Read the model definition and answer for the solid it produces. Units are mm, in the model's axes. A direction names the side the tool comes from. Coordinates: 2 decimals unless noted, no trailing zeros. Write each loop counter-clockwise with the first axis right and the second up, starting at its lowest first coordinate (ties: lowest second). Pieces come first, ordered by that corner, then holes.
(1) Section D-D on z = 3 is taken. Write down the section's boundary in (x, y), then the cut area to 3 significant figures.
(2) Which of the six approach directions +Z, -Z, +X, -X, +Y, -Y give full straight-line access (tool end or side, diameter ignored) to faces 1 (the flat face through (66.01, 25.51, 26.07)), 2 (the flat face through (-65.99, 25.49, 26.06)), 3 (the flat face through (-66.4, 2.74, 28.52))?
(3) Section A-A on y = 15 is taken. Write down the section's boundary in (x, z).
(4) Section C-C on z = 43.5 is taken. Write down the section's boundary in (x, y), then the cut area to 3 significant figures.
(5) Find the intervals of material crossed by probe 1 along X at (y, z) = (15, -10); probe 2 along Y at (x, z) = (-61, 7.5); probe 3 along Y at (x, z) = (-64.25, -5.5), in increasing order.
(6) Section B-B on x = -64.25 is taken. Write down the section's boundary in (y, z), then the cut area to 3 significant figures.
(7) Given pin 1 (5 mm diameter, centred on x = 43.5, y = 26.5, fed in from +Z); pin 2 (1 mm diameter, centred on y = 16.5, z = 40, fed in from -X); pin 3 (4 mm diameter, centred on x = -6, y = 14, fed in from +Z), each flat-ended and moving along its own axis, determine where each tip first touches the part or whether it passes through.
(8) The mould has two halves that part along X. Classify faces 4 (the flat face through (-66.54, 0.99, 23.92)), 5 (the flat face through (66.4, 27.24, 28.52)), 6 (the flat face through (62, 5.5, 19)), 7 (the cylindrical face through (59.492, 15.209, -7.556)): +X half, -X half, draft (parallel to the pull), parting line (faces both ways), or undercut.
from build123d import *

# Parameters (mm, degrees)
BOSS_EXTRUDE1_DEPTH     = 30
CUT_EXTRUDE2_DEPTH      = 100.544588
CUT_EXTRUDE2_DEPTH_BACK = 100.544588
SKETCH8_R               = 4.7625
SKETCH9_W               = 19
SKETCH9_H               = 5.5
BOSS_EXTRUDE3_DEPTH     = 59.75
CUT_EXTRUDE3_DEPTH      = 98.483973042
CUT_EXTRUDE3_DEPTH_BACK = 98.483973042
CHAMFER4_SIZE           = 2
FILLET2_R               = 2


with BuildPart() as part:
    # Sketch1 → Boss-Extrude1 (new body)
    with BuildSketch(Plane(origin=(0, 0, 0), x_dir=(1, 0, 0), z_dir=(0, 1, 0))):
        with BuildLine():
            Line((-54.75, -11.5), (-54.75, -56.25))
            Line((-54.75, -56.25), (-44.75, -56.25))
            ThreePointArc((-44.75, -56.25), (0, -11.5), (44.75, -56.25))
            Line((44.75, -56.25), (54.75, -56.25))
            Line((54.75, -56.25), (54.75, -11.5))
            Line((54.75, -11.5), (54.75, 3.5))
            Line((54.75, 3.5), (73.75, 3.5))
            Line((73.75, 3.5), (73.75, 11.5))
            Line((73.75, 11.5), (54.75, 11.5))
            Line((54.75, 11.5), (-54.75, 11.5))
            Line((-54.75, 11.5), (-73.75, 11.5))
            Line((-73.75, 11.5), (-73.75, 3.5))
            Line((-73.75, 3.5), (-54.75, 3.5))
            Line((-54.75, 3.5), (-54.75, -11.5))
        make_face()
    extrude(amount=BOSS_EXTRUDE1_DEPTH)

    # Sketch8 → Cut-Extrude2 (cut, two sides: drawn at the far end of the back side and taken through both)
    with BuildSketch(Plane.XY.offset(-3.5).offset(-CUT_EXTRUDE2_DEPTH_BACK)):
        with Locations((-64.25, 15)):
            Circle(SKETCH8_R)
        with Locations((64.25, 15)):
            Circle(SKETCH8_R)
    extrude(amount=CUT_EXTRUDE2_DEPTH + CUT_EXTRUDE2_DEPTH_BACK, mode=Mode.SUBTRACT)

    # Sketch9 → Boss-Extrude3 (add)
    with BuildSketch(Plane.XY.offset(-3.5)):
        with Locations((-64.25, 27.25)):
            Rectangle(SKETCH9_W, SKETCH9_H)
        with Locations((-64.25, 2.75)):
            Rectangle(SKETCH9_W, SKETCH9_H)
        with Locations((64.25, 27.25)):
            Rectangle(SKETCH9_W, SKETCH9_H)
        with Locations((64.25, 2.75)):
            Rectangle(SKETCH9_W, SKETCH9_H)
    extrude(amount=BOSS_EXTRUDE3_DEPTH)

    # Sketch10 → Cut-Extrude3 (cut, two sides: drawn at the far end of the back side and taken through both)
    with BuildSketch(Plane(origin=(0, 30, 0), x_dir=(1, 0, 0), z_dir=(0, 1, 0)).offset(-CUT_EXTRUDE3_DEPTH_BACK)):
        Polygon((-59.25, -56.25), (-73.75, 0), (-73.75, -56.25), align=None)
        Polygon((73.75, -56.25), (59.25, -56.25), (73.75, 0), align=None)
    extrude(amount=CUT_EXTRUDE3_DEPTH + CUT_EXTRUDE3_DEPTH_BACK, mode=Mode.SUBTRACT)

    # Chamfer4
    chamfer4_edges = [part.edges().sort_by_distance(p)[0] for p in [
        (-66.5, 24.5, 28.125),
    ]]
    chamfer(chamfer4_edges, length=CHAMFER4_SIZE)
    chamfer4_2_edges = [part.edges().sort_by_distance(p)[0] for p in [
        (-66.5, 5.5, 28.125),
    ]]
    chamfer(chamfer4_2_edges, length=CHAMFER4_SIZE)
    chamfer4_3_edges = [part.edges().sort_by_distance(p)[0] for p in [
        (-66.5, 0, 28.125),
    ]]
    chamfer(chamfer4_3_edges, length=CHAMFER4_SIZE)
    chamfer4_4_edges = [part.edges().sort_by_distance(p)[0] for p in [
        (66.5, 0, 28.125),
    ]]
    chamfer(chamfer4_4_edges, length=CHAMFER4_SIZE)
    chamfer4_5_edges = [part.edges().sort_by_distance(p)[0] for p in [
        (-66.5, 30, 28.125),
    ]]
    chamfer(chamfer4_5_edges, length=CHAMFER4_SIZE)
    chamfer4_6_edges = [part.edges().sort_by_distance(p)[0] for p in [
        (66.5, 30, 28.125),
    ]]
    chamfer(chamfer4_6_edges, length=CHAMFER4_SIZE)
    chamfer4_7_edges = [part.edges().sort_by_distance(p)[0] for p in [
        (66.5, 5.5, 28.125),
    ]]
    chamfer(chamfer4_7_edges, length=CHAMFER4_SIZE)
    chamfer4_8_edges = [part.edges().sort_by_distance(p)[0] for p in [
        (66.5, 24.5, 28.125),
    ]]
    chamfer(chamfer4_8_edges, length=CHAMFER4_SIZE)

    # Fillet2
    fillet2_edges = [part.edges().sort_by_distance(p)[0] for p in [
        (44.75, 15, 56.25),
        (-44.75, 15, 56.25),
    ]]
    fillet(fillet2_edges, radius=FILLET2_R)


solid = part.part
Response:
1. outline: (-72.98, 2) - (-70.91, 0) - (70.91, 0) - (72.98, 2) - (72.98, 3.5) - (70.91, 5.5) - (54.75, 5.5) - (54.75, 24.5) - (70.91, 24.5) - (72.98, 26.5) - (72.98, 28) - (70.91, 30) - (-70.91, 30) - (-72.98, 28) - (-72.98, 26.5) - (-70.91, 24.5) - (-54.75, 24.5) - (-54.75, 5.5) - (-70.91, 5.5) - (-72.98, 3.5) - close
1. area: 3,670 mm2
2. face 1: +Z, +X
2. face 2: +Z, -X
2. face 3: +Z, -X, +Y, -Y
3. outline: (-73.75, -11.5) - (-69.01, -11.5) - (-69.01, -3.5) - (-73.75, -3.5) - close; (-59.49, -11.5) - (59.49, -11.5) - (59.49, -3.5) - (54.75, -3.5) - (54.75, 56.25) - (46.71, 56.25) arc R2 ccw to (44.71, 54.34) arc R44.75 cw to (-44.71, 54.34) arc R2 ccw to (-46.71, 56.25) - (-54.75, 56.25) - (-54.75, -3.5) - (-59.49, -3.5) - close; (69.01, -11.5) - (73.75, -11.5) - (73.75, -3.5) - (69.01, -3.5) - close
4. outline: (-62.54, 2) - (-60.47, 0) - (-42.9, 0) - (-42.9, 30) - (-60.47, 30) - (-62.54, 28) - (-62.54, 26.5) - (-60.47, 24.5) - (-54.75, 24.5) - (-54.75, 5.5) - (-60.47, 5.5) - (-62.54, 3.5) - close; (42.9, 0) - (60.47, 0) - (62.54, 2) - (62.54, 3.5) - (60.47, 5.5) - (54.75, 5.5) - (54.75, 24.5) - (60.47, 24.5) - (62.54, 26.5) - (62.54, 28) - (60.47, 30) - (42.9, 30) - close
4. area: 866 mm2
5. probe 1: x = -73.75 to -69.01, -59.49 to 59.49, 69.01 to 73.75
5. probe 2: y = 0 to 5.5, 24.5 to 30
5. probe 3: y = 0 to 10.24, 19.76 to 30
6. outline: (0, -11.5) - (10.24, -11.5) - (10.24, -3.5) - (5.5, -3.5) - (5.5, 28.84) - (3.5, 36.85) - (2, 36.85) - (0, 28.84) - close; (19.76, -11.5) - (30, -11.5) - (30, 28.84) - (28, 36.85) - (26.5, 36.85) - (24.5, 28.84) - (24.5, -3.5) - (19.76, -3.5) - close
6. area: 576 mm2
7. pin 1: stops at z = 56.12
7. pin 2: stops at x = -54.75
7. pin 3: stops at z = 12.22
8. face 4: -X half
8. face 5: +X half
8. face 6: draft
8. face 7: undercut
